```python
from build123d import *

# Parameters (mm, degrees)
BOSS_EXTRUDE1_DEPTH = 6.35
SKETCH2_R           = 6.35
SKETCH2_R_2         = 3.175
BOSS_EXTRUDE2_DEPTH = 11.176
SKETCH3_R           = 3.175
CUT_EXTRUDE1_DEPTH  = 49.23960885


with BuildPart() as part:
    # Sketch1 → Boss-Extrude1 (new body)
    with BuildSketch(Plane.XY):
        with BuildLine():
            Line((15.670482603, -2.54), (33.813735094, -2.54))
            ThreePointArc((33.813735094, -2.54), (33.100172266, -7.361988656), (31.702602715, -12.03184367))
            ThreePointArc((31.702602715, -12.03184367), (16.146500506, -16.146500506), (12.03184367, -31.702602715))
            ThreePointArc((12.03184367, -31.702602715), (7.361988656, -33.100172266), (2.54, -33.813735094))
            Line((2.54, -33.813735094), (2.54, -15.670482603))
            ThreePointArc((2.54, -15.670482603), (0, -13.130482603), (-2.54, -15.670482603))
            Line((-2.54, -15.670482603), (-2.54, -33.813735094))
            ThreePointArc((-2.54, -33.813735094), (-7.361988656, -33.100172266), (-12.03184367, -31.702602715))
            ThreePointArc((-12.03184367, -31.702602715), (-16.146500506, -16.146500506), (-31.702602715, -12.03184367))
            ThreePointArc((-31.702602715, -12.03184367), (-33.100172266, -7.361988656), (-33.813735094, -2.54))
            Line((-33.813735094, -2.54), (-15.670482603, -2.54))
            ThreePointArc((-15.670482603, -2.54), (-13.130482603, 0), (-15.670482603, 2.54))
            Line((-15.670482603, 2.54), (-33.813735094, 2.54))
            ThreePointArc((-33.813735094, 2.54), (-33.100172266, 7.361988656), (-31.702602715, 12.03184367))
            ThreePointArc((-31.702602715, 12.03184367), (-16.146500506, 16.146500506), (-12.03184367, 31.702602715))
            ThreePointArc((-12.03184367, 31.702602715), (-7.361988656, 33.100172266), (-2.54, 33.813735094))
            Line((-2.54, 33.813735094), (-2.54, 15.670482603))
            ThreePointArc((-2.54, 15.670482603), (0, 13.130482603), (2.54, 15.670482603))
            Line((2.54, 15.670482603), (2.54, 33.813735094))
            ThreePointArc((2.54, 33.813735094), (7.361988656, 33.100172266), (12.03184367, 31.702602715))
            ThreePointArc((12.03184367, 31.702602715), (16.146500506, 16.146500506), (31.702602715, 12.03184367))
            ThreePointArc((31.702602715, 12.03184367), (33.100172266, 7.361988656), (33.813735094, 2.54))
            Line((33.813735094, 2.54), (15.670482603, 2.54))
            ThreePointArc((15.670482603, 2.54), (13.130482603, 0), (15.670482603, -2.54))
        make_face()
    extrude(amount=BOSS_EXTRUDE1_DEPTH)

    # Sketch2 → Boss-Extrude2 (add)
    with BuildSketch(Plane(origin=(0, 0, 0), x_dir=(-1, 0, 0), z_dir=(0, 0, -1))):
        Circle(SKETCH2_R)
        Circle(SKETCH2_R_2, mode=Mode.SUBTRACT)
    extrude(amount=-BOSS_EXTRUDE2_DEPTH)

    # Sketch3 → Cut-Extrude1 (cut, through all)
    with BuildSketch(Plane.XY.offset(6.35)):
        with Locations(Location((0, 0, 0), (0, 0, 180))):
            Circle(SKETCH3_R)
    extrude(amount=-CUT_EXTRUDE1_DEPTH, mode=Mode.SUBTRACT)


solid = part.part
```
Geometry check sheet. Reference: the model listing, model coordinates, mm. A direction names the side the tool comes from. Coordinates: 2 decimals unless noted, no trailing zeros. Order: outer loops, then holes, each group sorted by start corner. A loop starts at its lowest first (then second) coordinate and runs counter-clockwise, first axis right, second up. Notation, with made-up numbers: M 9.5,16 L 67.5,16 A33 cw 67.5,49 Z; hole C 42,-9 d11. An arc over 180 degrees is marked long. One line per question, with ' | ' between items. Start each with the question number.
Item 1: Cross-section at A-A on y = 0. Enter the section's corners in (x, z) (3 decimals).
Item 2: Material ranges on L1, parallel to X at y = 0, z = 5.75 (3 decimals); L2, parallel to Y at x = 0, z = 8.75 (3 decimals), recorded low to high. Write a range as [from, to].
Item 3: Draft check along Y on faces 1 (the cylindrical face through (-7.429, 33.085, 3.131)), 2 (the cylindrical face through (16.315, -15.981, 3.131)), 3 (the flat face through (2.54, -25, 3)), 4 (the cylindrical face through (-16.315, 15.981, 3.131)). Enter one of: pulls with the +Y half, pulls with the -Y half, needs draft (parallel to the pull), parting line crosses it, or undercut.
Item 4: Set-up check for faces 5 (the flat face through (-2.54, 25, 3)), 6 (the flat face through (25, 2.54, 3)), 7 (the flat face through (-2.54, -25, 3)), 8 (the flat face through (-25, -2.54, 3)): record each of +Z, -Z, +X, -X, +Y, -Y from which the full face is reachable in a straight line by a thin tool's end or side.
Item 5: Cross-section at B-B on x = 29.5. Enter the section's corners in (y, z), then the cut area to 3 significant figures.
Item 6: Gauge pin test, flat ends, axial feed: pin 1 (3 mm diameter, centred on y = 21, z = 2, fed in from +X); pin 2 (3 mm diameter, centred on y = 27, z = 4, fed in from -X); pin 3 (1.5 mm diameter, centred on x = 18.5, y = -12.5, fed in from -Z); pin 4 (1.9 mm diameter, centred on y = -29, z = 3.5, fed in from +X). Record the tip position at first contact, or that the pin passes through.
Item 7: Cross-section at C-C on z = 5.25. Enter the section's corners in (x, y) (3 decimals).
Findings:
1) outline: M -13.13,0 L -3.175,0 L -3.175,11.176 L -6.35,11.176 L -6.35,6.35 L -13.13,6.35 Z; M 3.175,0 L 13.13,0 L 13.13,6.35 L 6.35,6.35 L 6.35,11.176 L 3.175,11.176 Z
2) L1: x = [-13.13, -3.175], [3.175, 13.13] | L2: y = [-6.35, -3.175], [3.175, 6.35]
3) face 1: pulls with the +Y half | face 2: undercut | face 3: needs draft | face 4: undercut
4) face 5: +Z, -Z, +Y | face 6: +Z, -Z, +X | face 7: +Z, -Z, -Y | face 8: +Z, -Z, -X
5) outline: M -11.59,0 L -2.54,0 L -2.54,6.35 L -11.59,6.35 Z; M 2.54,0 L 11.59,0 L 11.59,6.35 L 2.54,6.35 Z | area: 115 mm²
6) pin 1: stops at x = 13.58 | pin 2: stops at x = -11.58 | pin 3: stops at z = 0 | pin 4: stops at x = 11.65
7) outline: M -33.814,-2.54 A33.909 ccw -31.703,-12.032 A16.002 cw -12.032,-31.703 A33.909 ccw -2.54,-33.814 L -2.54,-15.67 A2.54 cw 2.54,-15.67 L 2.54,-33.814 A33.909 ccw 12.032,-31.703 A16.002 cw 31.703,-12.032 A33.909 ccw 33.814,-2.54 L 15.67,-2.54 A2.54 cw 15.67,2.54 L 33.814,2.54 A33.909 ccw 31.703,12.032 A16.002 cw 12.032,31.703 A33.909 ccw 2.54,33.814 L 2.54,15.67 A2.54 cw -2.54,15.67 L -2.54,33.814 A33.909 ccw -12.032,31.703 A16.002 cw -31.703,12.032 A33.909 ccw -33.814,2.54 L -15.67,2.54 A2.54 cw -15.67,-2.54 Z; hole C 0,0 d6.35
